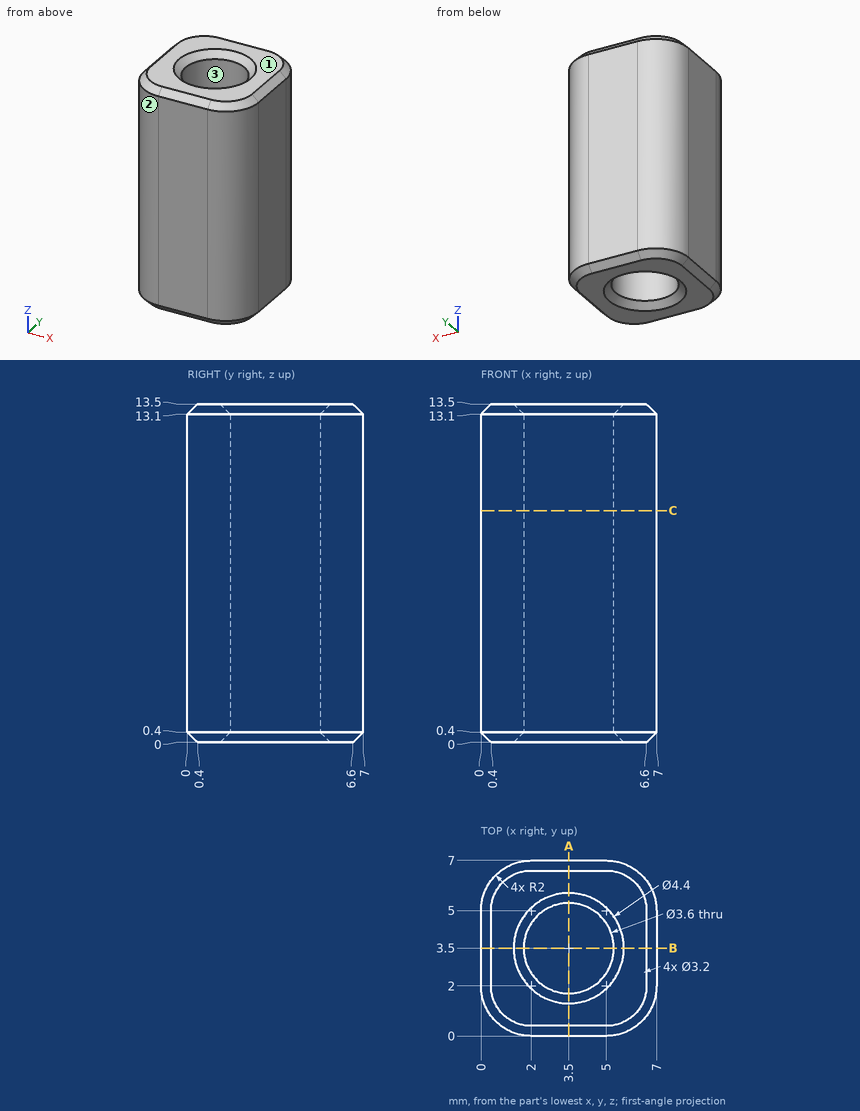
Drawing for the job (mm, zero at the part's lowest x, y, z). Round coordinates to 2 decimals unless told otherwise and drop trailing zeros. Write each loop counter-clockwise with the first axis right and the second up, starting at its lowest first coordinate (ties: lowest second). Pieces come first, ordered by that corner, then holes. Notation, with made-up numbers: (54.25, -17) - (88.25, -17) arc R32 cw to (88.25, 10) - close; hole circle Ø3 at (79, 11). An arc over 180 degrees is marked (long way). Use CSV: the item, a comma, the result in double quotes.
(1) Band-saw the part on A-A (x = 3.5). Write the cut outline in (y, z).
Response:
outline,"(0, 0.4) - (0.4, 0) - (1.3, 0) - (1.7, 0.4) - (1.7, 13.1) - (1.3, 13.5) - (0.4, 13.5) - (0, 13.1) - close; (5.3, 0.4) - (5.7, 0) - (6.6, 0) - (7, 0.4) - (7, 13.1) - (6.6, 13.5) - (5.7, 13.5) - (5.3, 13.1) - close"
(2) Mould opens along X. For the marked faces 1, 2 and 3 say: pulls with the +X half, pulls with the -X half, needs draft (parallel to the pull), parting line crosses it, or undercut.
Response:
face 1,"needs draft"
face 2,"pulls with the -X half"
face 3,"undercut"
(3) Band-saw the part on C-C (z = 9.25). Write the cut outline in (x, y), plus the area to 3 significant figures.
Response:
outline,"(0, 2) arc R2 ccw to (2, 0) - (5, 0) arc R2 ccw to (7, 2) - (7, 5) arc R2 ccw to (5, 7) - (2, 7) arc R2 ccw to (0, 5) - close; hole circle Ø3.6 at (3.5, 3.5)"
area,"35.4 mm²"
(4) Wall check: line 1 (Y direction, x = 3.5, z = 5.75); line 2 (Y direction, x = 2.5, z = 10); line 3 (X direction, y = 2.25, z = 4). Give the ranges that are in metal, low to high.
Response:
line 1,"0 to 1.7, 5.3 to 7"
line 2,"0 to 2, 5 to 7"
line 3,"0 to 2.2, 4.8 to 7"
